Work out the finished part from the listing and answer in its coordinate system (mm). Face numbers are marked on the shaded views. Round coordinates to 2 decimals unless told otherwise and drop trailing zeros. Write each loop counter-clockwise with the first axis right and the second up, starting at its lowest first coordinate (ties: lowest second). Pieces come first, ordered by that corner, then holes. Notation, with made-up numbers: M 23.5,-5.5 L 70.5,-5.5 A23 cw 70.5,30.5 Z; hole C 45,59 d8. An arc over 180 degrees is marked long. Answer in a Markdown table with one row per item.
```python
from build123d import *

# Parameters (mm, degrees)
BOSS_EXTRUDE1_DEPTH = 5
SKETCH2_R           = 2.5
SKETCH2_R_2         = 1.5
CUT_EXTRUDE1_DEPTH  = 10
FILLET2_R           = 5


# Some blends are built 0.0001 mm under size
with BuildPart() as part:
    # Sketch1 → Boss-Extrude1 (new body)
    with BuildSketch(Plane.XY):
        with BuildLine():
            ThreePointArc((0, -40), (28.284271247, -28.284271247), (40, 0))
            ThreePointArc((40, 0), (25.942500138, 30.446456059), (-6.349334329, 39.492859526))
            ThreePointArc((-6.349334329, 39.492859526), (5.815471714, 0.464499257), (0, -40))
        make_face()
    extrude(amount=BOSS_EXTRUDE1_DEPTH)

    # Sketch2 → Cut-Extrude1 (cut)
    with BuildSketch(Plane.XY.offset(5)):
        with Locations((15, -25)):
            Circle(SKETCH2_R)
        with Locations((27.5, 0)):
            Circle(SKETCH2_R_2)
        with Locations((15, 25)):
            Circle(SKETCH2_R_2)
    extrude(amount=-CUT_EXTRUDE1_DEPTH, mode=Mode.SUBTRACT)

    # Chamfer1
    # the kernel refuses this chamfer: 10, 7.744855577 mm, written as the material it takes off along each edge
    with BuildSketch(Plane(origin=(0, -40, -27.321942893), x_dir=(0.9956355834600147, 0.09332622861894702, 0), z_dir=(0, 0, 1))) as chamfer1_piece_1:
        with BuildLine():
            Line((7.46609829, 0), (4.150714585, 9.782810082))
            ThreePointArc((4.150714585, 9.782810082), (2.27411481, 4.969757663), (0, 0))
            ThreePointArc((0, 0), (3.797218814, -0.17452519), (7.46609829, 0))
        make_face()
    extrude(amount=59.643885786, mode=Mode.SUBTRACT)

    # Fillet2
    fillet2_edges = [part.edges().sort_by_distance(p)[0] for p in [
        (5.326559747, -34.587866421, 0),
        (5.24041299, 5.748958646, 0),
        (39.401767574, 6.892076033, 0),
    ]]
    fillet(fillet2_edges, radius=FILLET2_R - 0.0001)  # a hair under: the kernel refuses the full size


solid = part.part
```
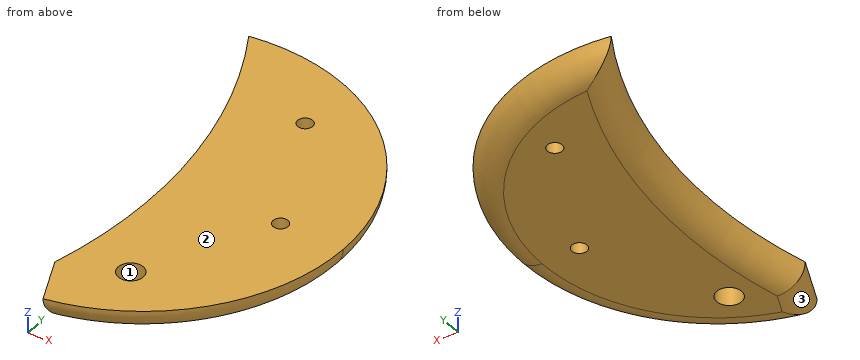
1. The part is cut by section B-B (x = 15). Count the separate pieces of the cut face and the enclosed holes in it, plus the area to 3 significant figures.
Calculated:
| item | result |
|---|---|
| separate pieces | 3 |
| enclosed holes | 0 |
| area | 319 mm² |
2. Given pin 1 (1.5 mm diameter, centred on y = -30, z = 4.5, fed in from -X); pin 2 (1 mm diameter, centred on y = 11, z = 1, fed in from -X); pin 3 (1.5 mm diameter, centred on x = 35, z = 4, fed in from -Y); pin 4 (2.5 mm diameter, centred on x = 15, y = 25, fed in from +Z), each flat-ended and moving along its own axis, determine where each tip first touches the part or whether it passes through.
Calculated:
| item | result |
|---|---|
| pin 1 | stops at x = 3.22 |
| pin 2 | stops at x = 5.81 |
| pin 3 | stops at y = -20.5 |
| pin 4 | passes through |
3. Determine the mould class of the marked faces 1, 2 and 3 for opening direction Y: released by +Y, released by -Y, zero draft, split by the parting line, or undercut.
Calculated:
| item | result |
|---|---|
| face 1 | undercut |
| face 2 | zero draft |
| face 3 | released by -Y |
4. Consider line 1 along Y through (x, z) = (15, 3.65); line 2 along Y through (x, z) = (15, 1.5); line 3 along X through (y, z) = (24.5, 3.45). Determine where each line is inside the solid, lowest interval first. Write a range as from..to.
Calculated:
| item | result |
|---|---|
| line 1 | y = -36.88..-27.5, -22.5..23.5, 26.5..36.88 |
| line 2 | y = -35.53..-27.5, -22.5..23.5, 26.5..35.53 |
| line 3 | x = 0.88..13.59, 16.41..31.31 |
5. The part is cut by section A-A (z = 2.9). Determine the outline of the cut face in (x, y), plus the area to 3 significant figures.
Calculated:
| item | result |
|---|---|
| outline | M -5.61,39.14 A93.11 cw 3.71,-29.83 L 7.71,-38.78 A39.54 ccw Z; hole C 15,-25 d5; hole C 15,25 d3; hole C 27.5,0 d3 |
| area | 2,120 mm² |
